For this review, take the finished solid that the model builds, in its own axes (mm). Face numbers are marked on the shaded views. A direction names the side the tool comes from. Coordinates: 2 decimals unless noted, no trailing zeros. Order: outer loops, then holes, each group sorted by start corner. A loop starts at its lowest first (then second) coordinate and runs counter-clockwise, first axis right, second up.
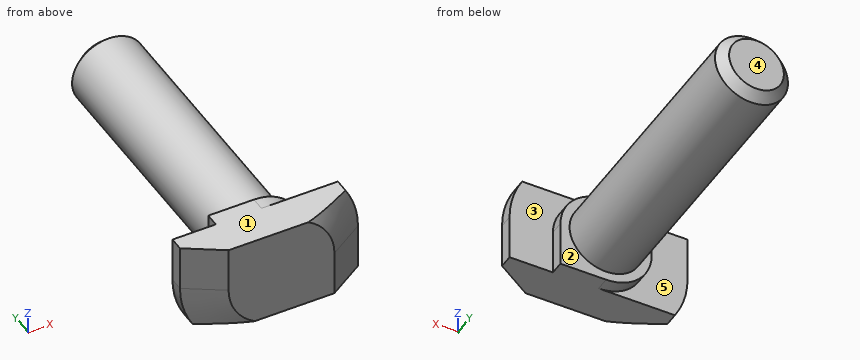
from build123d import *

# Parameters (mm, degrees)
EXTRUDE_1_DEPTH     = 5
CUT_EXTRUDE_1_DEPTH = 1.5
SKETCH_2_R          = 4
EXTRUDE_2_DEPTH     = 30
CUT_EXTRUDE_2_DEPTH = 5
CHAMFER_2_SIZE      = 1


with BuildPart() as part:
    # Эскиз1 → Бобышка-Вытянуть1 (new body, symmetric)
    with BuildSketch(Plane.XY):
        Polygon((9.75, 0), (-9.75, 0), (-9.75, 4), (-5, 4), (-5, 5.5), (5, 5.5), (5, 4), (9.75, 4), align=None)
    extrude(amount=EXTRUDE_1_DEPTH, both=True)

    # Эскиз3 → Вырез-Вытянуть1 (cut)
    with BuildSketch(Plane(origin=(0, 5.5, 0), x_dir=(1, 0, 0), z_dir=(0, 1, 0))):
        with BuildLine():
            Line((-5, 0), (-5, 5))
            Line((-5, 5), (0, 5))
            ThreePointArc((0, 5), (-3.535533906, 3.535533906), (-5, 0))
        make_face()
        with BuildLine():
            Line((0, -5), (5, -5))
            Line((5, -5), (5, 0))
            ThreePointArc((5, 0), (3.535533906, -3.535533906), (0, -5))
        make_face()
    extrude(amount=-CUT_EXTRUDE_1_DEPTH, mode=Mode.SUBTRACT)

    # Эскиз2 → Бобышка-Вытянуть2 (add)
    with BuildSketch(Plane(origin=(0, 5.5, 0), x_dir=(1, 0, 0), z_dir=(0, 1, 0))):
        with Locations(Location((0, 0, 0), (0, 0, 270))):  # turned: the seam where the file's is
            Circle(SKETCH_2_R)
    extrude(amount=EXTRUDE_2_DEPTH)

    # Эскиз4 → Вырез-Вытянуть2 (cut, through all)
    with BuildSketch(Plane(origin=(0, 4, 0), x_dir=(1, 0, 0), z_dir=(0, 1, 0))):
        with BuildLine():
            Line((-8.370334521, 5), (-9.75, 5))
            Line((-9.75, 5), (-9.75, 0))
            ThreePointArc((-9.75, 0), (-9.398756875, 2.59342808), (-8.370334521, 5))
        make_face()
        with BuildLine():
            Line((8.370334521, -5), (9.75, -5))
            Line((9.75, -5), (9.75, 0))
            ThreePointArc((9.75, 0), (9.398756875, -2.59342808), (8.370334521, -5))
        make_face()
    extrude(amount=-CUT_EXTRUDE_2_DEPTH, mode=Mode.SUBTRACT)

    # Вырез-По траектории1: sweep along a path in Эскиз6
    with BuildLine(Plane.XZ) as sweep_1_path:
        Line((0, -9.75), (9.75, -9.75))
        Line((9.75, -9.75), (9.75, 0))
        ThreePointArc((9.75, 0), (6.894291117, 6.894291117), (0, 9.75))
        Line((0, 9.75), (-9.75, 9.75))
        Line((-9.75, 9.75), (-9.75, 0))
        ThreePointArc((-9.75, 0), (-6.894291117, -6.894291117), (0, -9.75))
    # Эскиз5 → Вырез-По траектории1 (sweep, cut)
    with BuildSketch(Plane.XY.offset(5)):
        Polygon((-9.75, 2.5), (-5.8, 0), (-9.75, 0), align=None)
    sweep(path=sweep_1_path.line, transition=Transition.RIGHT, mode=Mode.SUBTRACT)

    # Фаска2
    chamfer_2_edges = [part.edges().sort_by_distance(p)[0] for p in [
        (0, 35.5, -4),
    ]]
    chamfer(chamfer_2_edges, length=CHAMFER_2_SIZE)


solid = part.part
1. Clearance check with flat-ended pins moving along their axes: pin 1 Ø1.5 at (y, z) = (15, -0.5) entering from -X; pin 2 Ø1.6 at (y, z) = (5, 3) entering from -X; pin 3 Ø0.8 at (y, z) = (5, -3) entering from +X; pin 4 Ø1 at (x, y) = (-7, 5.5) entering from +Z. State where each tip first meets the part, or that it passes through.
Answer below:
pin 1: stops at x = -4
pin 2: stops at x = -5
pin 3: stops at x = 5
pin 4: passes through
2. To check wall thickness, follow L1, parallel to Y at x = 4.5, z = 0.25; L2, parallel to X at y = 8, z = 0.25; L3, parallel to Y at x = -8, z = 1. State the ranges of each line that lie inside material, in increasing order.
Answer below:
L1: y = 0 to 5.5
L2: x = -3.99 to 3.99
L3: y = 1.39 to 4
3. Take a section at A-A, the plane y = 27. Give the boundary of the cut face in (x, z), plus the area to 3 significant figures.
Answer below:
outline: circle Ø8 at (0, 0)
area: 50.3 mm2
4. Machinability: for the marked faces 1, 2, 3, 4 and 5, which of the approach directions +Z, -Z, +X, -X, +Y, -Y give a long, thin tool a straight path to every point of the face, cutting with its end or side? Answer none if there is none.
Answer below:
face 1: +Z, +X, -X, +Y, -Y
face 2: +Y
face 3: +Z, +X, +Y
face 4: +Z, -Z, +X, -X, +Y
face 5: -Z, -X, +Y
